Source: three-view drawing plus pictorial views. Frame: mm from the lowest corner of the part. Coordinates: 2 decimals unless noted, no trailing zeros. Write each loop counter-clockwise with the first axis right and the second up, starting at its lowest first coordinate (ties: lowest second). Pieces come first, ordered by that corner, then holes. Notation, with made-up numbers: (-39.75, 23) - (16.25, 23) arc R9 cw to (16.25, 36) - close; hole circle Ø11 at (31.5, 84). An arc over 180 degrees is marked (long way). Put each result on its own line as item: value. Start each with the question number.
1. Cut plane C-C, the plane y = 12. Return loops of the section in (x, z).
2. Pin query (flat end, axial travel): pin 1 (2 mm diameter, centred on x = 4, y = 14, fed in from +Z); pin 2 (0.8 mm diameter, centred on x = 4, z = 14, fed in from +Y). Return the tip coordinate at first contact, or that it passes through.
3. Cut plane D-D, the plane x = 5.5. Return loops of the section in (y, z).
4. Cut plane B-B, the plane x = 3.75. Return loops of the section in (y, z).
5. Line query: line 1 (X direction, y = 14, z = 20.5); line 2 (Z direction, x = 3, y = 13.75); line 3 (Z direction, x = 4.75, y = 11.5). Output: solid intervals per line, ascending.
6. Cut plane A-A, the plane z = 10.5. Return loops of the section in (x, y).
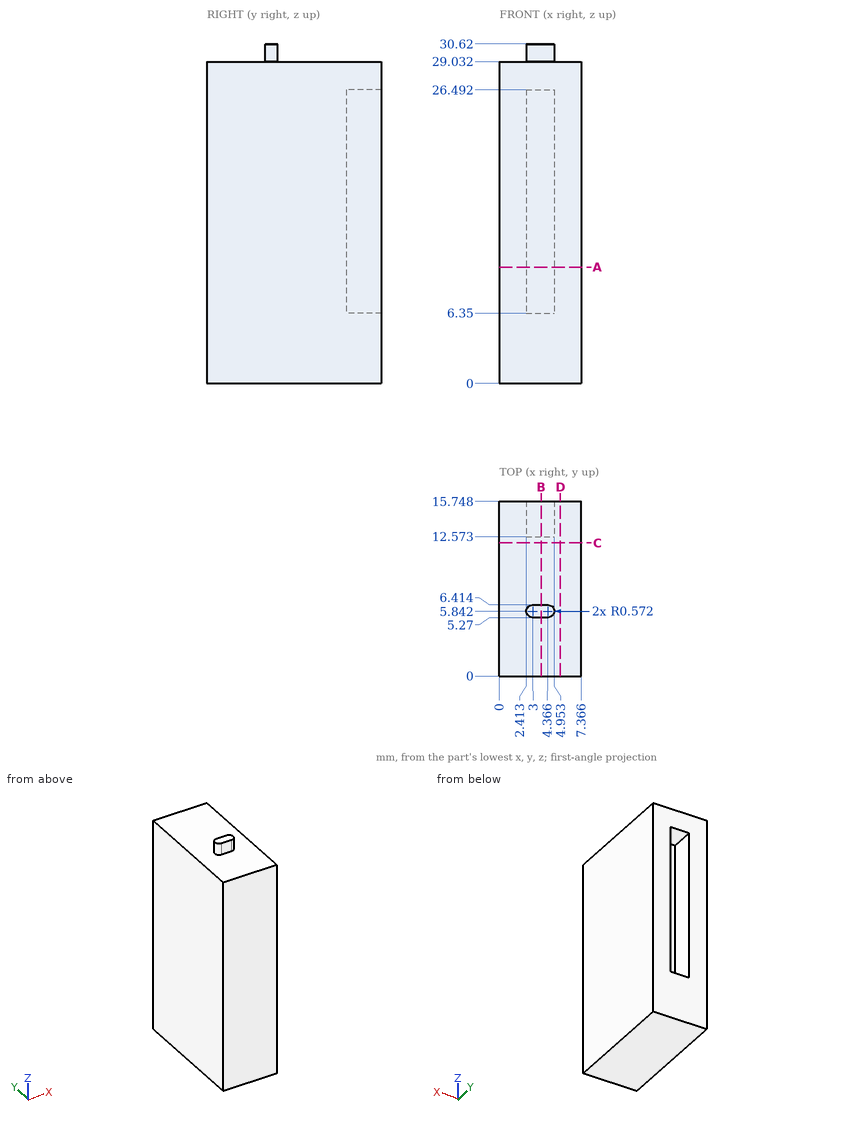
Report:
1. outline: (0, 0) - (7.37, 0) - (7.37, 29.03) - (0, 29.03) - close
2. pin 1: stops at z = 29.03
2. pin 2: stops at y = 12.57
3. outline: (0, 0) - (15.75, 0) - (15.75, 29.03) - (0, 29.03) - close
4. outline: (0, 0) - (15.75, 0) - (15.75, 6.35) - (12.57, 6.35) - (12.57, 26.49) - (15.75, 26.49) - (15.75, 29.03) - (6.41, 29.03) - (6.41, 30.62) - (5.27, 30.62) - (5.27, 29.03) - (0, 29.03) - close
5. line 1: x = 0 to 2.41, 4.95 to 7.37
5. line 2: z = 0 to 6.35, 26.49 to 29.03
5. line 3: z = 0 to 29.03
6. outline: (0, 0) - (7.37, 0) - (7.37, 15.75) - (4.95, 15.75) - (4.95, 12.57) - (2.41, 12.57) - (2.41, 15.75) - (0, 15.75) - close
